from build123d import *

# Parameters (mm, degrees)
CUT_EXTRUDE_1_DEPTH      = 4.5
CUT_EXTRUDE_1_DEPTH_BACK = 2.1


with BuildPart() as part:
    # Эскиз1 → Повернуть1 (revolve)
    with BuildSketch(Plane.XY):
        Polygon((-1.5, 24.5), (-1.5, 20), (4, 20), (4, 0), (5.5, 0), (5.5, 24.5), (2, 24.5), (2, 25.5), (0, 25.5), (0, 24.5), align=None)
    revolve(axis=Axis((-6.564956253, 0, 0), (1, 0, 0)))

    # Эскиз2 → Вырез-Вытянуть1 (cut, two sides)
    with BuildSketch(Plane(origin=(2, 0, 0), x_dir=(0, 0, -1), z_dir=(1, 0, 0))) as cut_extrude_1_sk:
        with BuildLine():
            ThreePointArc((-10.953795409, 23.027469816), (-22.083647797, 12.75), (-25.41927155, -2.027469816))
            Line((-25.41927155, -2.027469816), (-24.496248212, -0.428746497))
            ThreePointArc((-24.496248212, -0.428746497), (-21.217622393, 12.25), (-11.876818747, 21.428746497))
            Line((-11.876818747, 21.428746497), (-10.953795409, 23.027469816))
        make_face()
        with BuildLine():
            ThreePointArc((-11.876818747, 21.428746497), (-21.217622393, 12.25), (-24.496248212, -0.428746497))
            Line((-24.496248212, -0.428746497), (-11.876818747, 21.428746497))
        make_face()
        with BuildLine():
            Line((12.619429464, -21), (-12.619429464, -21))
            ThreePointArc((-12.619429464, -21), (0, -24.5), (12.619429464, -21))
        make_face()
        with BuildLine():
            Line((-12.619429464, -21), (-14.465476141, -21))
            ThreePointArc((-14.465476141, -21), (0, -25.5), (14.465476141, -21))
            Line((14.465476141, -21), (12.619429464, -21))
            ThreePointArc((12.619429464, -21), (0, -24.5), (-12.619429464, -21))
        make_face()
        with BuildLine():
            ThreePointArc((24.5, 0), (21.109619363, 12.435190804), (11.876818747, 21.428746497))
            Line((11.876818747, 21.428746497), (24.496248212, -0.428746497))
            ThreePointArc((24.496248212, -0.428746497), (24.499062035, -0.214381456), (24.5, 0))
        make_face()
        with BuildLine():
            ThreePointArc((25.5, 0), (21.558893558, 13.618520791), (10.953795409, 23.027469816))
            Line((10.953795409, 23.027469816), (11.876818747, 21.428746497))
            ThreePointArc((11.876818747, 21.428746497), (21.109619363, 12.435190804), (24.5, 0))
            ThreePointArc((24.5, 0), (24.499062035, -0.214381456), (24.496248212, -0.428746497))
            Line((24.496248212, -0.428746497), (25.41927155, -2.027469816))
            ThreePointArc((25.41927155, -2.027469816), (25.479809895, -1.014538188), (25.5, 0))
        make_face()
    extrude(amount=CUT_EXTRUDE_1_DEPTH, mode=Mode.SUBTRACT)
    extrude(cut_extrude_1_sk.sketch, amount=-CUT_EXTRUDE_1_DEPTH_BACK, mode=Mode.SUBTRACT)


solid = part.part
Geometry check sheet. Reference: the model listing, model coordinates, mm. A direction names the side the tool comes from. Give positions to 0.01 mm unless a question says otherwise; leave off trailing zeros. Write each loop counter-clockwise with the first axis right and the second up, starting at its lowest first coordinate (ties: lowest second). Pieces come first, ordered by that corner, then holes.
1) Cross-section at B-B (z = 0). Record the boundary of the cut face in (x, y), plus the area to 3 significant figures.
Values follow:
outline: (-1.5, -24.5) - (-0.1, -24.5) - (-0.1, -21) - (5.5, -21) - (5.5, 24.5) - (2, 24.5) - (2, 25.5) - (0, 25.5) - (0, 24.5) - (-1.5, 24.5) - (-1.5, 20) - (4, 20) - (4, -20) - (-1.5, -20) - close
area: 105 mm2
2) Go/stop test with flat-tipped pins: pin 1 Ø10 at (y, z) = (9.5, -19.5) entering from +X; pin 2 Ø3 at (x, y) = (4.5, 5) entering from -Z; pin 3 Ø1 at (y, z) = (-23.5, -0.5) entering from +X; pin 4 Ø12 at (y, z) = (0.5, -0.5) entering from -X. Record where each tip stops, or that it passes through.
Values follow:
pin 1: stops at x = 5.5
pin 2: stops at z = -22.23
pin 3: stops at x = -0.1
pin 4: stops at x = 4
3) Cross-section at D-D (z = 9). Record the boundary of the cut face in (x, y), plus the area to 3 significant figures.
Values follow:
outline: (-1.5, -22.79) - (-0.1, -22.79) - (-0.1, -21) - (5.5, -21) - (5.5, 22.79) - (2, 22.79) - (2, 23.86) - (0, 23.86) - (0, 22.79) - (-1.5, 22.79) - (-1.5, 17.86) - (4, 17.86) - (4, -17.86) - (-1.5, -17.86) - close
area: 115 mm2
4) Thickness scan on line 1 (X direction, y = -2, z = 19); line 2 (X direction, y = 10.5, z = -20.5); line 3 (Z direction, x = 0.5, y = 0). Record the ranges inside material, lowest first.
Values follow:
line 1: x = 4 to 5.5
line 2: x = -1.5 to -0.1
line 3: z = -24.25 to -20, 20 to 24.25
5) Cross-section at C-C (y = 5.5). Record the boundary of the cut face in (x, z).
Values follow:
outline: (-1.5, -23.87) - (-0.1, -23.87) - (-0.1, -21.07) - (5.5, -21.07) - (5.5, 21.07) - (-0.1, 21.07) - (-0.1, 23.87) - (-1.5, 23.87) - (-1.5, 19.23) - (4, 19.23) - (4, -19.23) - (-1.5, -19.23) - close
6) Set-up check for faces 1 (the face through (-0.1, 11, -19)), 2 (the face through (3.73, -12.4, -21.13)), 3 (the face through (0, 25, 1)), 4 (the face through (2, 25, 0)), 5 (the face through (3.726, -12.099, 21.304)): record each of +Z, -Z, +X, -X, +Y, -Y from which the full face is reachable in a straight line by a thin tool's end or side.
Values follow:
face 1: -Z, +X, +Y
face 2: -Z, +X, -Y
face 3: -X, +Y
face 4: +X, +Y
face 5: +Z, +X, -Y
7) Cross-section at A-A (x = 0.75). Record the boundary of the cut face in (y, z).
Values follow:
outline: (-21, -14.47) arc R25.5 ccw to (-2.03, -25.42) - (23.03, -10.95) arc R25.5 ccw to (23.03, 10.95) - (-2.03, 25.42) arc R25.5 ccw to (-21, 14.47) - close; hole circle Ø40 at (0, 0)
8) Release check for a two-part mould opening along Z. For faces 6 (the face through (1.288, -4.336, -19.524)), 7 (the face through (3, -21, 0)), 8 (the face through (1, 25.5, -0.2)) record: released by +Z, released by -Z, zero draft, split by the parting line, or undercut.
Values follow:
face 6: undercut
face 7: zero draft
face 8: split by the parting line
